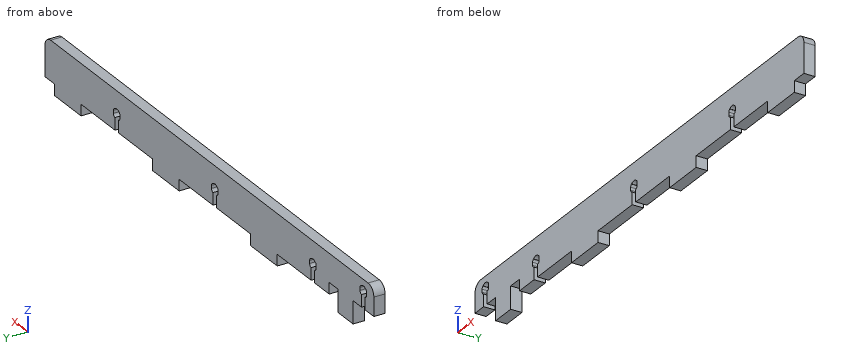
from build123d import *

# Parameters (mm, degrees)
SALIENTE_EXTRUIR1_DEPTH = 6


with BuildPart() as part:
    # Croquis1 → Saliente-Extruir1 (new body)
    with BuildSketch(Plane(origin=(0, 0, 0), x_dir=(1, 0, 0), z_dir=(0, 1, 0))):
        with BuildLine():
            Line((-122.476621199, -5.742358079), (-114.926621199, -5.742358079))
            Line((-114.926621199, -5.742358079), (-114.926621199, -12.242583321))
            ThreePointArc((-114.926621199, -12.242583321), (-115.851225833, -12.770672857), (-116.216958829, -13.770678689))
            Line((-116.216958829, -13.770678689), (-116.216958829, -15.320678689))
            ThreePointArc((-116.216958829, -15.320678689), (-116.028261999, -16.061862661), (-115.508115372, -16.622583321))
            Line((-115.508115372, -16.622583321), (-115.33887044, -16.622583321))
            ThreePointArc((-115.33887044, -16.622583321), (-113.376621199, -17.435593306), (-111.414371957, -16.622583321))
            Line((-111.414371957, -16.622583321), (-111.245127025, -16.622583321))
            ThreePointArc((-111.245127025, -16.622583321), (-110.724980398, -16.061862661), (-110.536283568, -15.320678689))
            Line((-110.536283568, -15.320678689), (-110.536283568, -13.770678689))
            ThreePointArc((-110.536283568, -13.770678689), (-110.902016564, -12.770672857), (-111.826621199, -12.242583321))
            Line((-111.826621199, -12.242583321), (-111.826621199, -5.742358079))
            Line((-111.826621199, -5.742358079), (-104.476621199, -5.742358079))
            Line((-104.476621199, -5.742358079), (-104.476621199, 6.257641921))
            Line((-104.476621199, 6.257641921), (-91.476621199, 6.257641921))
            Line((-91.476621199, 6.257641921), (-91.476621199, -5.742358079))
            Line((-91.476621199, -5.742358079), (-83.776621199, -5.742358079))
            Line((-83.776621199, -5.742358079), (-83.776621199, 0.257641921))
            Line((-83.776621199, 0.257641921), (-71.226621199, 0.257641921))
            Line((-71.226621199, 0.257641921), (-71.226621199, -6.242583321))
            ThreePointArc((-71.226621199, -6.242583321), (-72.151225833, -6.770672857), (-72.516958829, -7.770678689))
            Line((-72.516958829, -7.770678689), (-72.516958829, -9.320678689))
            ThreePointArc((-72.516958829, -9.320678689), (-72.328261999, -10.061862661), (-71.808115372, -10.622583321))
            Line((-71.808115372, -10.622583321), (-71.63887044, -10.622583321))
            ThreePointArc((-71.63887044, -10.622583321), (-69.676621199, -11.435593306), (-67.714371957, -10.622583321))
            Line((-67.714371957, -10.622583321), (-67.545127025, -10.622583321))
            ThreePointArc((-67.545127025, -10.622583321), (-67.024980398, -10.061862661), (-66.836283568, -9.320678689))
            Line((-66.836283568, -9.320678689), (-66.836283568, -7.770678689))
            ThreePointArc((-66.836283568, -7.770678689), (-67.202016564, -6.770672857), (-68.126621199, -6.242583321))
            Line((-68.126621199, -6.242583321), (-68.126621199, 0.257641921))
            Line((-68.126621199, 0.257641921), (-38.776621199, 0.257641921))
            Line((-38.776621199, 0.257641921), (-38.776621199, 6.257641921))
            Line((-38.776621199, 6.257641921), (-15.776621199, 6.257641921))
            Line((-15.776621199, 6.257641921), (-15.776621199, 0.257641921))
            Line((-15.776621199, 0.257641921), (13.773378801, 0.257641921))
            Line((13.773378801, 0.257641921), (13.773378801, -6.242583321))
            ThreePointArc((13.773378801, -6.242583321), (12.848774167, -6.770672857), (12.483041171, -7.770678689))
            Line((12.483041171, -7.770678689), (12.483041171, -9.320678689))
            ThreePointArc((12.483041171, -9.320678689), (12.671738001, -10.061862661), (13.191884628, -10.622583321))
            Line((13.191884628, -10.622583321), (13.36112956, -10.622583321))
            ThreePointArc((13.36112956, -10.622583321), (15.323378801, -11.435593306), (17.285628043, -10.622583321))
            Line((17.285628043, -10.622583321), (17.454872975, -10.622583321))
            ThreePointArc((17.454872975, -10.622583321), (17.975019602, -10.061862661), (18.163716432, -9.320678689))
            Line((18.163716432, -9.320678689), (18.163716432, -7.770678689))
            ThreePointArc((18.163716432, -7.770678689), (17.797983436, -6.770672857), (16.873378801, -6.242583321))
            Line((16.873378801, -6.242583321), (16.873378801, 0.257641921))
            Line((16.873378801, 0.257641921), (46.223378801, 0.257641921))
            Line((46.223378801, 0.257641921), (46.223378801, 6.257641921))
            Line((46.223378801, 6.257641921), (69.223378801, 6.257641921))
            Line((69.223378801, 6.257641921), (69.223378801, 0.257641921))
            Line((69.223378801, 0.257641921), (98.773378801, 0.257641921))
            Line((98.773378801, 0.257641921), (98.773378801, -6.242583321))
            ThreePointArc((98.773378801, -6.242583321), (97.848774167, -6.770672857), (97.483041171, -7.770678689))
            Line((97.483041171, -7.770678689), (97.483041171, -9.320678689))
            ThreePointArc((97.483041171, -9.320678689), (97.671738001, -10.061862661), (98.191884628, -10.622583321))
            Line((98.191884628, -10.622583321), (98.36112956, -10.622583321))
            ThreePointArc((98.36112956, -10.622583321), (100.323378801, -11.435593306), (102.285628043, -10.622583321))
            Line((102.285628043, -10.622583321), (102.454872975, -10.622583321))
            ThreePointArc((102.454872975, -10.622583321), (102.975019602, -10.061862661), (103.163716432, -9.320678689))
            Line((103.163716432, -9.320678689), (103.163716432, -7.770678689))
            ThreePointArc((103.163716432, -7.770678689), (102.797983436, -6.770672857), (101.873378801, -6.242583321))
            Line((101.873378801, -6.242583321), (101.873378801, 0.257641921))
            Line((101.873378801, 0.257641921), (131.223378801, 0.257641921))
            Line((131.223378801, 0.257641921), (131.223378801, 6.257641921))
            Line((131.223378801, 6.257641921), (154.223378801, 6.257641921))
            Line((154.223378801, 6.257641921), (154.223378801, 0.257641921))
            Line((154.223378801, 0.257641921), (162.523378801, 0.257641921))
            Line((162.523378801, 0.257641921), (162.523378801, -0.742358079))
            Line((162.523378801, -0.742358079), (162.523378801, -15.742358079))
            ThreePointArc((162.523378801, -15.742358079), (161.058912707, -19.277891985), (157.523378801, -20.742358079))
            Line((157.523378801, -20.742358079), (-117.476621199, -20.742358079))
            ThreePointArc((-117.476621199, -20.742358079), (-121.012155104, -19.277891985), (-122.476621199, -15.742358079))
            Line((-122.476621199, -15.742358079), (-122.476621199, -5.742358079))
        make_face()
    extrude(amount=SALIENTE_EXTRUIR1_DEPTH)


solid = part.part
Read the model definition and answer for the solid it produces. Units are mm, in the model's axes. Coordinates: 2 decimals unless noted, no trailing zeros. Loops run counter-clockwise (first coordinate to the right, second up) from the corner with the lowest first, then second, coordinate; pieces in that order, holes last.
Q1. Each of these flat-tipped pins is pushed along its axis until it touches: pin 1 Ø1.8 at (x, y) = (115, 2) entering from -Z; pin 2 Ø3 at (x, y) = (-108.5, 3) entering from -Z; pin 3 Ø1.8 at (y, z) = (1.5, 3.5) entering from -X; pin 4 Ø6 at (x, z) = (8, 7) entering from -Y. Where does it stop, or does it pass through?
Q2. Consider probe 1 along X at (y, z) = (0.6, 0.5); probe 2 along X at (y, z) = (1.1, -3); probe 3 along X at (y, z) = (2.9, 7.25). Determine where each line is inside the solid, lowest interval first.
Q3. The part is cut by section A-A on z = 3. Write down the section's boundary in (x, y).
Q4. The part is cut by section B-B on x = -1.5. Write down the section's boundary in (y, z), and give its area (3 significant figures).
Results below:
1. pin 1: stops at z = -0.26
1. pin 2: stops at z = 5.74
1. pin 3: stops at x = -104.48
1. pin 4: stops at y = 0
2. probe 1: x = -104.48 to -91.48, -83.78 to -71.23, -68.13 to 13.77, 16.87 to 98.77, 101.87 to 162.52
2. probe 2: x = -104.48 to -91.48, -38.78 to -15.78, 46.22 to 69.22, 131.22 to 154.22
2. probe 3: x = -122.48 to -114.93, -111.83 to -72.43, -66.93 to 12.57, 18.07 to 97.57, 103.07 to 162.52
3. outline: (-104.48, 0) - (-91.48, 0) - (-91.48, 6) - (-104.48, 6) - close; (-83.78, 0) - (-71.23, 0) - (-71.23, 6) - (-83.78, 6) - close; (-68.13, 0) - (13.77, 0) - (13.77, 6) - (-68.13, 6) - close; (16.87, 0) - (98.77, 0) - (98.77, 6) - (16.87, 6) - close; (101.87, 0) - (162.52, 0) - (162.52, 6) - (101.87, 6) - close
4. outline: (0, -0.26) - (6, -0.26) - (6, 20.74) - (0, 20.74) - close
4. area: 126 mm2
